Read the model definition and answer for the solid it produces. Units are mm, in the model's axes. A direction names the side the tool comes from. Coordinates: 2 decimals unless noted, no trailing zeros. Loops run counter-clockwise (first coordinate to the right, second up) from the corner with the lowest first, then second, coordinate; pieces in that order, holes last. Notation, with made-up numbers: (24, 84) - (42, 84) arc R34 cw to (42, 118) - close; hole circle Ø11 at (30, -3.75). An arc over 180 degrees is marked (long way). Use one line per item in the form item = value. Start each with the question number.
1) Each of these flat-tipped pins is pushed along its axis until it touches: P1, Ø24, axis at x = 99.5, z = 13, coming from the +Y side; P2, Ø5, axis at x = -29.5, y = -123.5, coming from the +Z side; P3, Ø6, axis at x = 18.5, z = 43.5, coming from the -Y side; P4, Ø12, axis at y = -47.5, z = 29, coming from the +X side. Where does it stop, or does it pass through?
2) A cutting plane is placed at C-C (x = 19.5). State how many separate pieces and enclosed holes the cut face has, and give its area (3 significant figures).
3) A cutting plane is placed at A-A (z = 47). Give the vertices of the cut face in (x, y).
4) A cutting plane is placed at D-D (z = 4). Give the vertices of the cut face in (x, y), and give its area (3 significant figures).
5) Consider line 1 (Y direction, x = -16.5, z = 13); line 2 (Y direction, x = 97.5, z = 15); line 3 (Z direction, x = 47, y = -85.5). Determine where each line is inside the solid, lowest interval first.
6) The mould has two halves that part along X. Classify faces 1 (the face through (105.747, -42.971, 8.555)), 2 (the face through (13.963, -113.775, 12.747)), 3 (the face through (-33.17, 27.84, 2.85)), 4 (the face through (-26, -124, 20)): released by +X, released by -X, zero draft, split by the parting line, or undercut.
7) Which of the six approach directions +Z, -Z, +X, -X, +Y, -Y give full straight-line access (tool end or side, diameter ignored) to faces 5 (the face through (-36.18, 28, 15)), 6 (the face through (16.575, -111.164, 51.654)), 7 (the face through (38.8, -84.01, 29.58)), 8 (the face through (-16.18, 28, 30)), 9 (the face through (77, -38.041, 30))?
8) A cutting plane is placed at B-B (z = 35). Give the vertices of the cut face in (x, y), and give its area (3 significant figures).
from build123d import *

# Parameters (mm, degrees)
SALIENTE_EXTRUIR1_DEPTH    = 60
CROQUIS3_W                 = 40
CROQUIS3_H                 = 20
CORTAR_EXTRUIR1_DEPTH      = 46
CROQUIS4_R                 = 15
CORTAR_EXTRUIR5_DEPTH      = 57
CORTAR_EXTRUIR6_DEPTH      = 16
CORTAR_EXTRUIR6_DEPTH_BACK = 19
CROQUIS12_R                = 7.5
CROQUIS12_R_2              = 15
REDONDEO2_R                = 10
REDONDEO3_R                = 30
CROQUIS13_R                = 15
CORTAR_EXTRUIR7_DEPTH      = 82
REDONDEO4_R                = 30
CROQUIS14_W                = 20
CROQUIS14_H                = 20
CORTAR_EXTRUIR8_DEPTH      = 156
CORTAR_EXTRUIR9_DEPTH      = 37
CORTAR_EXTRUIR9_DEPTH_BACK = 54
CROQUIS16_R                = 7.5
CROQUIS16_R_2              = 15
REDONDEO5_R                = 10


with BuildPart() as part:
    # Croquis2 → Saliente-Extruir1 (new body)
    with BuildSketch(Plane.XY):
        Polygon((-36.180131723, 22.907142857), (3.819868277, 22.907142857), (74.767829948, -48.040818814), (114.767829948, -48.040818814), (114.767829948, -38.040818814), (74.767829948, -38.040818814), (3.819868277, 32.907142857), (-36.180131723, 32.907142857), align=None)
    saliente_extruir1 = extrude(amount=SALIENTE_EXTRUIR1_DEPTH)

    # Croquis3 → Cortar-Extruir1 (cut)
    with BuildSketch(Plane(origin=(0, 0, 0), x_dir=(1, 0, 0), z_dir=(0, 1, 0))):
        with Locations((-36.180131723, -30)):
            Rectangle(CROQUIS3_W, CROQUIS3_H)
    extrude(amount=CORTAR_EXTRUIR1_DEPTH, mode=Mode.SUBTRACT)

    # Croquis4 → Cortar-Extruir5 (cut)
    with BuildSketch(Plane(origin=(0, 0, 0), x_dir=(1, 0, 0), z_dir=(0, 1, 0))):
        with Locations(Location((94.767829948, -30, 0), (0, 0, 270))):
            Circle(CROQUIS4_R)
    extrude(amount=-CORTAR_EXTRUIR5_DEPTH, mode=Mode.SUBTRACT)

    # Croquis12 → Cortar-Extruir6 (cut, two sides: drawn at the far end of the back side and taken through both)
    with BuildSketch(Plane(origin=(18.363505567, 18.363505567, 0), x_dir=(0, 0, -1), z_dir=(0.7071067811865486, 0.7071067811865465, 0)).offset(-CORTAR_EXTRUIR6_DEPTH_BACK)):
        with Locations(Location((-15, -4.516083302, 0), (0, 0, 270))):
            Circle(CROQUIS12_R)
        with Locations(Location((-45, -4.516083302, 0), (0, 0, 270))):
            Circle(CROQUIS12_R)
        with Locations(Location((-30, -54.683868112, 0), (0, 0, 270))):
            Circle(CROQUIS12_R_2)
    extrude(amount=CORTAR_EXTRUIR6_DEPTH + CORTAR_EXTRUIR6_DEPTH_BACK, mode=Mode.SUBTRACT)

    # Redondeo2
    redondeo2_edges = [part.edges().sort_by_distance(p)[0] for p in [
        (-36.180131723, 27.907142857, 0),
        (-36.180131723, 27.907142857, 60),
    ]]
    fillet(redondeo2_edges, radius=REDONDEO2_R)

    # Redondeo3
    redondeo3_edges = [part.edges().sort_by_distance(p)[0] for p in [
        (114.767829948, -43.040818814, 60),
        (114.767829948, -43.040818814, 0),
    ]]
    fillet(redondeo3_edges, radius=REDONDEO3_R - 0.0001)  # a hair under: the kernel refuses the full size

    # Simetría1: Saliente-Extruir1 across plane
    add(saliente_extruir1.mirror(Plane(origin=(114.767829948, -48.040818814, 60), x_dir=(0, 0, 1), z_dir=(0, 1, 0))))

    # Croquis13 → Cortar-Extruir7 (cut)
    with BuildSketch(Plane(origin=(0, 0, 0), x_dir=(1, 0, 0), z_dir=(0, 1, 0))):
        with Locations((94.767829948, -30)):
            Circle(CROQUIS13_R)
    extrude(amount=-CORTAR_EXTRUIR7_DEPTH, mode=Mode.SUBTRACT)

    # Redondeo4
    redondeo4_edges = [part.edges().sort_by_distance(p)[0] for p in [
        (114.767829948, -53.040818814, 0),
        (114.767829948, -53.040818814, 60),
    ]]
    fillet(redondeo4_edges, radius=REDONDEO4_R - 0.0001)  # a hair under: the kernel refuses the full size

    # Croquis14 → Cortar-Extruir8 (cut)
    with BuildSketch(Plane(origin=(0, 0, 0), x_dir=(1, 0, 0), z_dir=(0, 1, 0))):
        with Locations((-26.180131723, -30)):
            Rectangle(CROQUIS14_W, CROQUIS14_H)
    extrude(amount=-CORTAR_EXTRUIR8_DEPTH, mode=Mode.SUBTRACT)

    # Croquis16 → Cortar-Extruir9 (cut, two sides: drawn at the far end of the back side and taken through both)
    with BuildSketch(Plane(origin=(66.404324381, -66.404324381, 0), x_dir=(0, 0, -1), z_dir=(0.7071067811865486, -0.7071067811865465, 0)).offset(-CORTAR_EXTRUIR9_DEPTH_BACK)):
        with Locations(Location((-45, -63.423894212, 0), (0, 0, 270))):
            Circle(CROQUIS16_R)
        with Locations(Location((-15, -63.423894212, 0), (0, 0, 270))):
            Circle(CROQUIS16_R)
        with Locations(Location((-30, -13.256109403, 0), (0, 0, 270))):
            Circle(CROQUIS16_R_2)
    extrude(amount=CORTAR_EXTRUIR9_DEPTH + CORTAR_EXTRUIR9_DEPTH_BACK, mode=Mode.SUBTRACT)

    # Redondeo5
    redondeo5_edges = [part.edges().sort_by_distance(p)[0] for p in [
        (-36.180131723, -123.988780485, 60),
        (-36.180131723, -123.988780485, 0),
    ]]
    fillet(redondeo5_edges, radius=REDONDEO5_R)


solid = part.part
Found:
q1.P1 = -38.04
q1.P2 = 59.97
q1.P3 = -117.31
q1.P4 = 114.77
q2.separate_pieces = 6
q2.enclosed_holes = 0
q2.area = 625 mm^2
q3.outline = (-36.18, -128.99) - (3.82, -128.99) - (16.45, -116.36) - (11.45, -111.36) - (3.82, -118.99) - (-36.18, -118.99) - close; (-36.18, 22.91) - (3.82, 22.91) - (11.45, 15.28) - (16.45, 20.28) - (3.82, 32.91) - (-36.18, 32.91) - close; (21.67, -101.14) - (26.67, -106.14) - (74.77, -58.04) - (109.49, -58.04) - (109.49, -38.04) - (74.77, -38.04) - (26.67, 10.06) - (21.67, 5.06) - (74.77, -48.04) - close
q4.outline = (-34.18, -128.99) - (3.82, -128.99) - (74.77, -58.04) - (99.73, -58.04) - (99.73, -38.04) - (74.77, -38.04) - (3.82, 32.91) - (-34.18, 32.91) - (-34.18, 22.91) - (3.82, 22.91) - (74.77, -48.04) - (3.82, -118.99) - (-34.18, -118.99) - close
q4.area = 2,680 mm^2
q5.line_1 = -128.99 to -118.99, 22.91 to 32.91
q5.line_2 = -58.04 to -38.04
q5.line_3 = 0 to 24.53, 35.47 to 60
q6.face_1 = released by +X
q6.face_2 = undercut
q6.face_3 = released by -X
q6.face_4 = zero draft
q7.face_5 = +Z, -Z, -X, +Y, -Y
q7.face_6 = none
q7.face_7 = +Z, -Z, -X
q7.face_8 = -X, +Y, -Y
q7.face_9 = +Z, -Z, +X, +Y
q8.outline = (-16.18, -128.99) - (3.82, -128.99) - (47.03, -85.78) - (42.03, -80.78) - (3.82, -118.99) - (-16.18, -118.99) - close; (-16.18, 22.91) - (3.82, 22.91) - (42.03, -15.3) - (47.03, -10.3) - (3.82, 32.91) - (-16.18, 32.91) - close; (62.03, -60.78) - (67.03, -65.78) - (74.77, -58.04) - (80.63, -58.04) - (80.63, -38.04) - (74.77, -38.04) - (67.03, -30.3) - (62.03, -35.3) - (74.77, -48.04) - close; (108.91, -58.04) - (114.35, -58.04) - (114.35, -38.04) - (108.91, -38.04) - close
q8.area = 1,640 mm^2
